from build123d import *

# Parameters (mm, degrees)
CROQUIS1_R              = 75
SALIENTE_EXTRUIR1_DEPTH = 4
CROQUIS3_R              = 75
CROQUIS3_R_2            = 70
SALIENTE_EXTRUIR2_DEPTH = 4
SALIENTE_EXTRUIR3_DEPTH = 1
CROQUIS2_R              = 2.5
CORTAR_EXTRUIR1_DEPTH   = 2
CROQUIS4_R              = 25
CORTAR_EXTRUIR2_DEPTH   = 6


with BuildPart() as part:
    # Croquis1 → Saliente-Extruir1 (new body)
    with BuildSketch(Plane(origin=(0, 0, 0), x_dir=(1, 0, 0), z_dir=(0, 1, 0))):
        with Locations(Location((0, 0, 0), (0, 0, 270))):
            Circle(CROQUIS1_R)
    extrude(amount=SALIENTE_EXTRUIR1_DEPTH)

    # Croquis3 → Saliente-Extruir2 (add)
    with BuildSketch(Plane(origin=(0, 4, 0), x_dir=(1, 0, 0), z_dir=(0, 1, 0))):
        with Locations(Location((0, 0, 0), (0, 0, 270))):
            Circle(CROQUIS3_R)
        with Locations(Location((0, 0, 0), (0, 0, 270))):
            Circle(CROQUIS3_R_2, mode=Mode.SUBTRACT)
    extrude(amount=SALIENTE_EXTRUIR2_DEPTH)

    # Croquis7 → Saliente-Extruir3 (add)
    with BuildSketch(Plane(origin=(0, 4, 0), x_dir=(1, 0, 0), z_dir=(0, 1, 0))):
        Polygon((0.75, -1.810660172), (51.618795027, -52.679455198), (52.679455198, -51.618795027), (1.810660172, -0.75), (73.75, -0.75), (73.75, 0.75), (1.810660172, 0.75), (52.679455198, 51.618795027), (51.618795027, 52.679455198), (0.75, 1.810660172), (0.75, 73.75), (-0.75, 73.75), (-0.75, 1.810660172), (-51.618795027, 52.679455198), (-52.679455198, 51.618795027), (-1.810660172, 0.75), (-73.75, 0.75), (-73.75, -0.75), (-1.810660172, -0.75), (-52.679455198, -51.618795027), (-51.618795027, -52.679455198), (-0.75, -1.810660172), (-0.75, -73.75), (0.75, -73.75), align=None)
    extrude(amount=SALIENTE_EXTRUIR3_DEPTH)

    # Croquis2 → Cortar-Extruir1 (cut)
    with BuildSketch(Plane.XZ):
        with Locations(Location((-60, 0, 0), (0, 0, 270))):
            Circle(CROQUIS2_R)
        with Locations(Location((-42.426406871, 42.426406871, 0), (0, 0, 270))):
            Circle(CROQUIS2_R)
        with Locations(Location((0, 60, 0), (0, 0, 270))):
            Circle(CROQUIS2_R)
        with Locations(Location((42.426406871, 42.426406871, 0), (0, 0, 270))):
            Circle(CROQUIS2_R)
        with Locations(Location((60, 0, 0), (0, 0, 270))):
            Circle(CROQUIS2_R)
        with Locations(Location((42.426406871, -42.426406871, 0), (0, 0, 270))):
            Circle(CROQUIS2_R)
        with Locations(Location((0, -60, 0), (0, 0, 270))):
            Circle(CROQUIS2_R)
        with Locations(Location((-42.426406871, -42.426406871, 0), (0, 0, 270))):
            Circle(CROQUIS2_R)
    extrude(amount=-CORTAR_EXTRUIR1_DEPTH, mode=Mode.SUBTRACT)

    # Croquis4 → Cortar-Extruir2 (cut)
    with BuildSketch(Plane.XZ):
        with Locations(Location((0, 0, 0), (0, 0, 270))):
            Circle(CROQUIS4_R)
    extrude(amount=-CORTAR_EXTRUIR2_DEPTH, mode=Mode.SUBTRACT)


solid = part.part
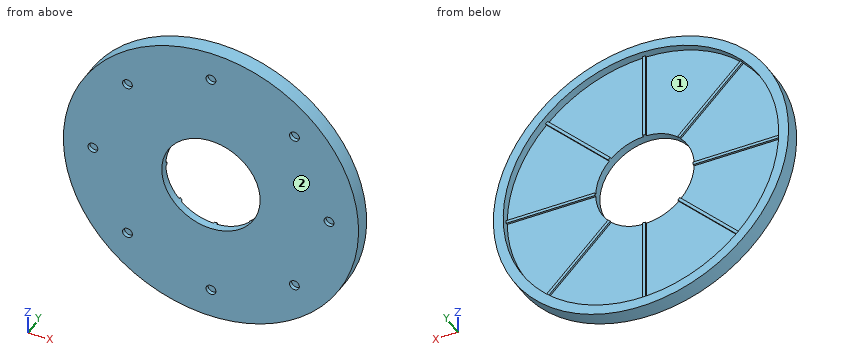
The listing builds one solid part. Answer for the finished solid, in the listing's coordinates (mm). Face numbers are marked on the shaded views. Coordinates: 2 decimals unless noted, no trailing zeros. Order: outer loops, then holes, each group sorted by start corner. A loop starts at its lowest first (then second) coordinate and runs counter-clockwise, first axis right, second up.
Q1. Given P1, Ø2.5, axis at x = -59.5, z = 0, coming from the -Y side; P2, Ø1.5, axis at x = 46.5, z = 41, coming from the +Y side; P3, Ø0.8, axis at y = 4.5, z = 40, coming from the +X side, each flat-ended and moving along its own axis, determine where each tip first touches the part or whether it passes through.
Q2. A cutting plane is placed at D-D, the plane x = -60. Write down the section's boundary in (y, z).
Q3. A cutting plane is placed at A-A, the plane z = -12. Write down the section's boundary in (x, y), and give its area (3 significant figures).
Q4. A cutting plane is placed at C-C, the plane z = 37. Write down the section's boundary in (x, y), and give its area (3 significant figures).
Q5. For a pull along Z with two mould halves and no side action, classify the marked faces 1 and 2 as pulls with the +Z half, pulls with the -Z half, needs draft (parallel to the pull), parting line crosses it, or undercut.
Q6. Consider line 1 (X direction, y = 7.5, z = 1); line 2 (X direction, y = 3.5, z = 0.5) (3 decimals); line 3 (Z direction, x = -32.5, y = 4.75). Determine where each line is inside the solid, lowest interval first.
Q7. A cutting plane is placed at B-B, the plane x = -36.5. Write down the section's boundary in (y, z), and give its area (3 significant figures).
Answers follow:
1. P1: stops at y = 2
1. P2: stops at y = 4
1. P3: stops at x = 63.69
2. outline: (0, -45) - (8, -45) - (8, -36.06) - (4, -36.06) - (4, -0.75) - (5, -0.75) - (5, 0.75) - (4, 0.75) - (4, 36.06) - (8, 36.06) - (8, 45) - (0, 45) - (0, 2.5) - (2, 2.5) - (2, -2.5) - (0, -2.5) - close
3. outline: (-74.03, 0) - (-21.93, 0) - (-21.93, 4) - (-68.96, 4) - (-68.96, 8) - (-74.03, 8) - close; (21.93, 0) - (74.03, 0) - (74.03, 8) - (68.96, 8) - (68.96, 4) - (21.93, 4) - close
3. area: 457 mm2
4. outline: (-65.24, 0) - (65.24, 0) - (65.24, 8) - (59.42, 8) - (59.42, 4) - (38.06, 4) - (38.06, 5) - (35.94, 5) - (35.94, 4) - (0.75, 4) - (0.75, 5) - (-0.75, 5) - (-0.75, 4) - (-35.94, 4) - (-35.94, 5) - (-38.06, 5) - (-38.06, 4) - (-59.42, 4) - (-59.42, 8) - (-65.24, 8) - close
4. area: 574 mm2
5. face 1: undercut
5. face 2: needs draft
6. line 1: x = -74.99 to -69.99, 69.99 to 74.99
6. line 2: x = -74.998 to -24.995, 24.995 to 74.998
6. line 3: z = -67.59 to -62, -33.56 to -31.44, -0.75 to 0.75, 31.44 to 33.56, 62 to 67.59
7. outline: (0, -65.52) - (8, -65.52) - (8, -59.73) - (4, -59.73) - (4, -37.56) - (5, -37.56) - (5, -35.44) - (4, -35.44) - (4, -0.75) - (5, -0.75) - (5, 0.75) - (4, 0.75) - (4, 35.44) - (5, 35.44) - (5, 37.56) - (4, 37.56) - (4, 59.73) - (8, 59.73) - (8, 65.52) - (0, 65.52) - close
7. area: 576 mm2
